Model file for the job. Use its own axes, mm. Face numbers are marked on the shaded views. A direction names the side the tool comes from. Give positions to 0.01 mm unless a question says otherwise; leave off trailing zeros. Loops run counter-clockwise (first coordinate to the right, second up) from the corner with the lowest first, then second, coordinate; pieces in that order, holes last. Notation, with made-up numbers: (-35.5, 55) -> (-23.5, 55) arc R19 ccw to (-23.5, 78) -> close; hole circle Ø3 at (34, 86). An arc over 180 degrees is marked (long way). Use CSV: the item, a comma, the result in double quotes. Start each with the question number.
(1) Drill centre lines: probe 1 along Z at (x, y) = (4.5, 21.25); probe 2 along Y at (x, z) = (7, 5.75); probe 3 along Z at (x, y) = (6.75, 8.25). Where is each one in solid material? Low to high.
(2) Pull direction Z, two halves, no side cores. Call the marked faces 1, 2, 3 and 4: pulls with the +Z half, pulls with the -Z half, needs draft (parallel to the pull), parting line crosses it, or undercut.
(3) Cut at D-D on z = 12.25. Write the cut outline in (x, y), then the cut area to 3 significant figures.
(4) Cut at A-A on x = 7. Write the cut outline in (y, z), then the cut area to 3 significant figures.
(5) Flat gauge pins, fed straight in: pin 1 (9 mm diameter, centred on x = 9.5, y = 6, fed in from +Z); pin 2 (3.5 mm diameter, centred on y = 18.5, z = 12.5, fed in from -X). Where does each tip first touch, or does it go through?
(6) Cut at B-B on z = 9.5. Write the cut outline in (x, y), then the cut area to 3 significant figures.
(7) 3-axis set-ups, long thin cutter, end or side, ignore diameter. For the marked faces 5, 6, 7 and 8: which of +Z, -Z, +X, -X, +Y, -Y reach the whole face in a straight line?
(8) Cut at C-C on y = 19.25. Write the cut outline in (x, z).
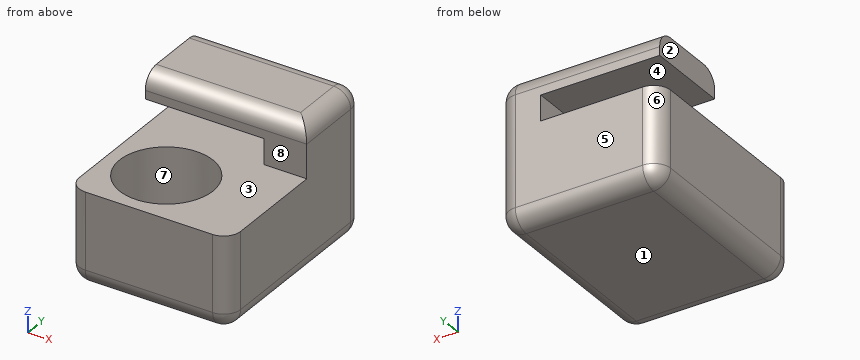
from build123d import *

# Parameters (mm, degrees)
CYLINDER_R     = 5.5
CYLINDER_DEPTH = 10
BOX001_W       = 5
BOX001_H       = 10
BOX001_DEPTH   = 3
BOX002_W       = 19
BOX002_H       = 10
BOX002_DEPTH   = 3
BOX_W          = 19
BOX_H          = 24
BOX_DEPTH      = 11
FILLET_R       = 2


with BuildPart() as magnet_hole:
    # Cylinder → Cylinder (new body)
    with BuildSketch(Plane(origin=(7, 7, 1), x_dir=(1, 0, 0), z_dir=(0, 0, 1))):
        Circle(CYLINDER_R)
    extrude(amount=CYLINDER_DEPTH)


with BuildPart() as cube001:
    # Box001 → Box001 (new body)
    with BuildSketch(Plane(origin=(14, 14, 11), x_dir=(1, 0, 0), z_dir=(0, 0, 1))):
        with Locations((2.5, 5)):
            Rectangle(BOX001_W, BOX001_H)
    extrude(amount=BOX001_DEPTH)


with BuildPart() as cube002:
    # Box002 → Box002 (new body)
    with BuildSketch(Plane(origin=(0, 14, 14), x_dir=(1, 0, 0), z_dir=(0, 0, 1))):
        with Locations((9.5, 5)):
            Rectangle(BOX002_W, BOX002_H)
    extrude(amount=BOX002_DEPTH)


with BuildPart() as fillet_body:
    # Box → Box (new body)
    with BuildSketch(Plane.XY):
        with Locations((9.5, 12)):
            Rectangle(BOX_W, BOX_H)
    extrude(amount=BOX_DEPTH)

    # Fusion: union Cube001, Cube002
    add(cube001.part)
    add(cube002.part)

    # Cut: cut Magnet Hole
    add(magnet_hole.part, mode=Mode.SUBTRACT)

    # Fillet
    fillet_edges = [fillet_body.edges().sort_by_distance(p)[0] for p in [
        (0, 0, 5.5),
        (0, 24, 5.5),
        (0, 12, 0),
        (9.5, 0, 0),
        (19, 0, 5.5),
        (9.5, 24, 0),
        (19, 24, 5.5),
        (19, 12, 0),
        (19, 24, 12.5),
        (9.5, 14, 17),
        (19, 24, 15.5),
        (9.5, 24, 17),
        (19, 19, 17),
    ]]
    fillet(fillet_edges, radius=FILLET_R)


solid = fillet_body.part
Check result:
1,probe 1,"0 to 11, 14 to 17"
1,probe 2,"0 to 1.5, 12.5 to 24"
1,probe 3,"0 to 1"
2,face 1,"pulls with the -Z half"
2,face 2,"needs draft"
2,face 3,"undercut"
2,face 4,"undercut"
3,outline,"(14, 14) -> (19, 14) -> (19, 22) arc R2 ccw to (17, 24) -> (14, 24) -> close"
3,area,"49.1 mm²"
4,outline,"(0, 2) arc R2 ccw to (2, 0) -> (22, 0) arc R2 ccw to (24, 2) -> (24, 11) -> (12.5, 11) -> (12.5, 1) -> (1.5, 1) -> (1.5, 11) -> (0, 11) -> close; (14, 14) -> (24, 14) -> (24, 15) arc R2 ccw to (22, 17) -> (16, 17) arc R2 ccw to (14, 15) -> close"
4,area,"181 mm²"
5,pin 1,"z = 11"
5,pin 2,"x = 0"
6,outline,"(0, 2) arc R2 ccw to (2, 0) -> (17, 0) arc R2 ccw to (19, 2) -> (19, 22) arc R2 ccw to (17, 24) -> (2, 24) arc R2 ccw to (0, 22) -> close; hole circle Ø11 at (7, 7)"
6,area,"358 mm²"
7,face 5,"+Z, -Z, +X, -X, +Y"
7,face 6,"-Z, -X, +Y"
7,face 7,"+Z"
7,face 8,"+Z, +X, -X, -Y"
8,outline,"(0, 2) arc R2 ccw to (2, 0) -> (17, 0) arc R2 ccw to (19, 2) -> (19, 15) arc R2 ccw to (17, 17) -> (0, 17) -> (0, 14) -> (14, 14) -> (14, 11) -> (0, 11) -> close"
